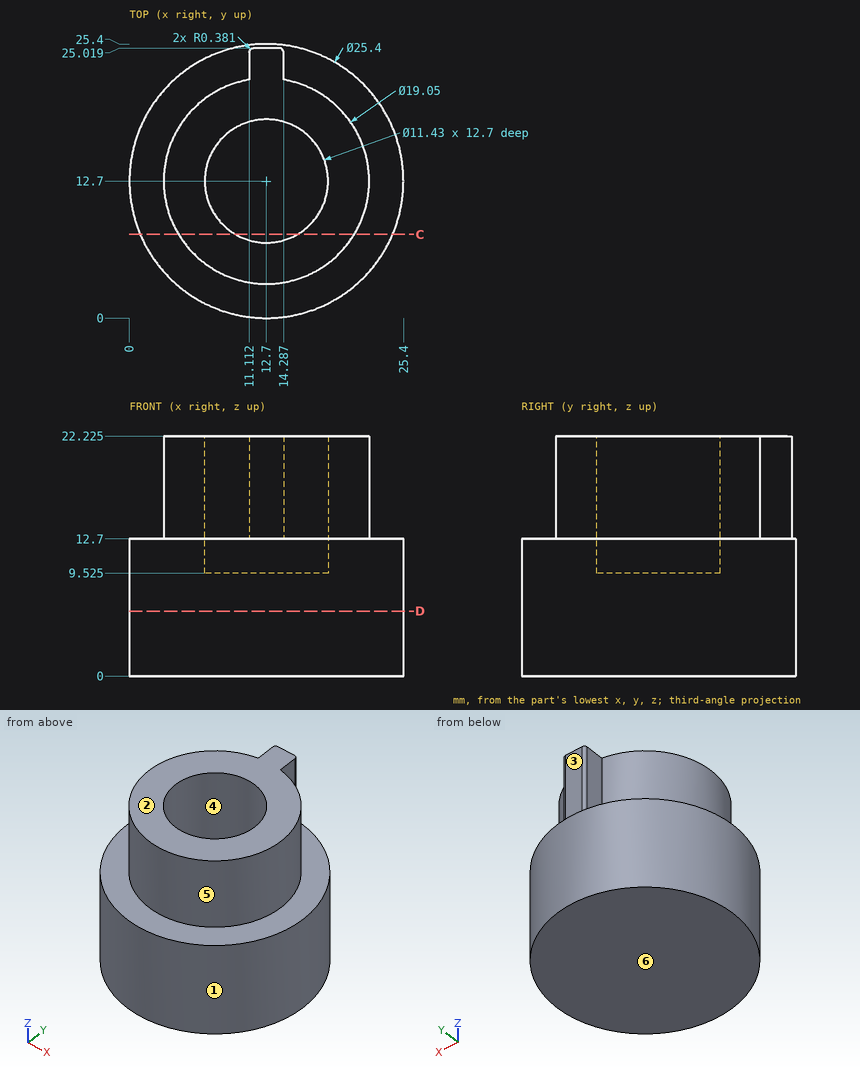
Source: three-view drawing plus pictorial views. Frame: mm from the lowest corner of the part. A direction names the side the tool comes from. Round coordinates to 2 decimals unless told otherwise and drop trailing zeros. Order: outer loops, then holes, each group sorted by start corner. A loop starts at its lowest first (then second) coordinate and runs counter-clockwise, first axis right, second up. Notation, with made-up numbers: M 66.25,54 L 74.25,54 A17 ccw 74.25,59 Z; hole C 64.5,76 d11. An arc over 180 degrees is marked long. One line per item, written item: value.
(1) Cut plane C-C (y = 7.75). Return the cut outline in (x, z) (1 decimal).
Result sheet:
outline: M 1,0 L 24.4,0 L 24.4,12.7 L 20.8,12.7 L 20.8,22.2 L 15.6,22.2 L 15.6,9.5 L 9.8,9.5 L 9.8,22.2 L 4.6,22.2 L 4.6,12.7 L 1,12.7 Z
(2) Line query: probe 1 along Y at (x, z) = (12.7, 14) (1 decimal); probe 2 along Z at (x, y) = (21.75, 5.75); probe 3 along X at (y, z) = (15, 17.5) (1 decimal). Output: solid intervals per line, ascending. Write a range as [from, to].
Result sheet:
probe 1: [3.2, 7], [18.4, 25]
probe 2: [0, 12.7]
probe 3: [3.5, 7.5], [17.9, 21.9]
(3) Pin query (flat end, axial travel): P1, Ø2, axis at x = 18.5, z = 17, coming from the +Y side; P2, Ø6, axis at x = 9.5, z = 14, coming from the -Y side; P3, Ø1.3, axis at y = 23.5, z = 19, coming from the +X side. Return the tip coordinate at first contact, or that it passes through.
Result sheet:
P1: y = 20.93
P2: y = 0.01
P3: x = 14.29
(4) Pull-direction query (Y, two-part tool) for the marked faces 1, 2, 3 and 4; classes: pulls with the +Y half, pulls with the -Y half, needs draft (parallel to the pull), parting line crosses it, or undercut.
Result sheet:
face 1: parting line crosses it
face 2: needs draft
face 3: pulls with the +Y half
face 4: undercut
(5) Cut plane D-D (z = 6). Return the cut outline in (x, y).
Result sheet:
outline: C 12.7,12.7 d25.4
(6) Reachability of the marked faces 5 and 6 from +Z, -Z, +X, -X, +Y, -Y: full face, straight path, thin tool, end or side. Return the list, or none.
Result sheet:
face 5: +Z
face 6: -Z, +X, -X, +Y, -Y
